Autodesk Inventor part; units mm, degrees
ref_plane "YZ Plane" through (0, 0, 0) normal (1, 0, 0) x (0, 1, 0)
ref_plane "XZ Plane" through (0, 0, 0) normal (0, 1, 0) x (-1, 0, 0)
ref_plane "XY Plane" through (0, 0, 0) normal (0, 0, 1) x (1, 0, 0)
ref_plane "Arbeitsebene1" through (-10.2983, 3.243, -1) normal (0, 0, -1) x (-1, 0, 0)
sketch "Skizze1" plane through (-10.2983, 3.243, -1) normal (0, 0, -1) x (-1, 0, 0)
  line L0 (2.7017, 34.757) -> (-23.2983, 34.757)
  line L1 (-23.2983, 34.757) -> (-23.2983, -41.243)
  line L2 (-23.2983, -41.243) -> (2.7017, -41.243)
  line L3 (2.7017, -41.243) -> (2.7017, 34.757)
  line L4 (3.7017, -42.243) -> (-24.2983, -42.243)
  line L5 (-24.2983, -42.243) -> (-24.2983, 35.757)
  line L6 (-24.2983, 35.757) -> (3.7017, 35.757)
  line L7 (3.7017, 35.757) -> (3.7017, -42.243)
  line L8 (7.7017, -46.243) -> (-28.2983, -46.243)
  line L9 (-28.2983, -46.243) -> (-28.2983, 39.757)
  line L10 (-28.2983, 39.757) -> (7.7017, 39.757)
  line L11 (7.7017, 39.757) -> (7.7017, -46.243)
  point P0 (-10.2983, -3.243)
  dimension "d1" = 4
  dimension "d39" = 36
extrude "Extrusion1" add sketch "Skizze1" along normal blind 3 contours L8 L9 L10 L11
sketch "Skizze2" plane through (-10.2983, 3.243, -1) normal (0, 0, 1) x (1, 0, 0)
  line L0 (24.2983, 35.757) -> (24.2983, -42.243)
  line L1 (24.2983, -42.243) -> (-3.7017, -42.243)
  line L2 (-3.7017, -42.243) -> (-3.7017, 35.757)
  line L3 (-3.7017, 35.757) -> (24.2983, 35.757)
  line L4 (-7.7017, -46.243) -> (28.2983, -46.243)
  line L5 (28.2983, -46.243) -> (28.2983, 39.757)
  line L6 (28.2983, 39.757) -> (-7.7017, 39.757)
  line L7 (-7.7017, 39.757) -> (-7.7017, -46.243)
  line L8 (22.2983, 33.757) -> (22.2983, -40.243)
  line L9 (22.2983, -40.243) -> (-1.7017, -40.243)
  line L10 (-1.7017, -40.243) -> (-1.7017, 33.757)
  line L11 (-1.7017, 33.757) -> (22.2983, 33.757)
  line L12 (21.2983, -39.243) -> (21.2983, 32.757)
  line L13 (21.2983, 32.757) -> (-0.7017, 32.757)
  line L14 (-0.7017, 32.757) -> (-0.7017, -39.243)
  line L15 (-0.7017, -39.243) -> (21.2983, -39.243)
  point P0 (10.2983, -3.243)
  dimension "d4" = 2
  dimension "d45" = 1
extrude "Extrusion2" add sketch "Skizze2" along normal blind 1 contours L0 L1 L2 L3 | L7 L6 L5 L4 | L8 L9 L10 L11
ref_plane "Arbeitsebene2" through (-18, -43, -2.5) normal (0, -1, 0) x (1, 0, 0)
sketch "Skizze9" plane through (-18, -43, -4) normal (-1, 0, 0) x (0, 0, 1)
  line L0 (0, 86) -> (4, 86)
  line L1 (0, 0) -> (0, 86)
  line L2 (4, 0) -> (0, 0)
  line L3 (4, 86) -> (4, 0)
  line L4 (4, 0) -> (3, 0)
  line L5 (3, 0) -> (3, 86)
  line L6 (3, 86) -> (4, 86)
  line L7 (4, 86) -> (4, 0)
  line L8 (4, 0) -> (3, 86) construction
  line L9 (3, 0) -> (4, 86) construction
  dimension "d27" = 1
extrude "Extrusion9" add sketch "Skizze9" along normal blind 3 contours L0 L3 L2 L5
sketch "Skizze10" plane through (18, -43, -4) normal (1, 0, 0) x (0, 0, -1)
  line L0 (-3, 86) -> (-3, 0)
  line L1 (-3, 0) -> (-4, 0)
  line L2 (-4, 0) -> (-4, 86)
  line L3 (-4, 86) -> (-3, 86)
  point P0 (-4, 43)
extrude "Extrusion10" add sketch "Skizze10" along normal blind 3
sketch "Skizze11" plane through (-10.2983, 3.243, 0) normal (0, 0, 1) x (1, 0, 0)
  line L0 (22.2983, -40.243) -> (-1.7017, -40.243)
  line L1 (-1.7017, -40.243) -> (-1.7017, 33.757)
  line L2 (-1.7017, 33.757) -> (22.2983, 33.757)
  line L3 (22.2983, 33.757) -> (22.2983, -40.243)
  line L4 (31.2983, 39.757) -> (-9.4351, 39.757)
  line L5 (-9.4351, 39.757) -> (-9.4351, 59.757)
  line L6 (-9.4351, 59.757) -> (31.2983, 59.757)
  line L7 (31.2983, 59.757) -> (31.2983, 39.757)
  line L8 (28.2983, 42.757) -> (-6.4351, 42.757)
  line L9 (-6.4351, 42.757) -> (-6.4351, 56.757)
  line L10 (-6.4351, 56.757) -> (28.2983, 56.757)
  line L11 (28.2983, 56.757) -> (28.2983, 42.757)
  point P0 (10.2983, -3.243)
  dimension "d32" = 20
  dimension "d33" = 3
extrude "Extrusion11" add sketch "Skizze11" against normal up to surface (4 mm away) contours L4 L5 L6 L7
sketch "Skizze12" plane through (-10.2983, 3.243, 0) normal (0, 0, 1) x (1, 0, 0)
  line L0 (28.2983, 56.757) -> (28.2983, 42.757)
  line L1 (28.2983, 42.757) -> (-6.4351, 42.757)
  line L2 (-6.4351, 42.757) -> (-6.4351, 56.757)
  line L3 (-6.4351, 56.757) -> (28.2983, 56.757)
  line L4 (31.2983, -46.243) -> (31.2983, 59.757)
  line L5 (31.2983, 59.757) -> (-9.4351, 59.757)
  line L6 (-9.4351, 59.757) -> (-9.4351, 39.757)
  line L7 (35.2983, 40.5388) -> (-14.7017, 40.5388)
  line L8 (-14.7017, 40.5388) -> (-14.7017, 42.757)
  line L9 (-14.7017, 42.757) -> (35.2983, 42.757)
  line L10 (35.2983, 42.757) -> (35.2983, 40.5388)
  line L11 (35.2983, 40.5388) -> (-14.7017, 42.757) construction
  line L12 (-14.7017, 40.5388) -> (35.2983, 42.757) construction
  line L13 (31.2983, -46.243) -> (-10.7017, -46.243)
  line L14 (-10.7017, 39.757) -> (-9.4351, 39.757)
  line L15 (-10.7017, -46.243) -> (-10.7017, 39.757)
  point P0 (10.2983, -3.243)
  point P1 (10.2983, 41.6479)
  dimension "d36" = 50
extrude "Extrusion12" add sketch "Skizze12" against normal blind 10 contours L9 L4 L7 L6 L1 | L9 L10 L7 L4 | L6 L7 L8 L9
sketch "Skizze13" plane through (-10.2983, 3.243, -4) normal (0, 0, -1) x (-1, 0, 0)
  line L0 (-24.2983, -42.243) -> (-24.2983, 35.757)
  line L1 (-24.2983, 35.757) -> (3.7017, 35.757)
  line L2 (3.7017, 35.757) -> (3.7017, -42.243)
  line L3 (3.7017, -42.243) -> (-24.2983, -42.243)
  line L4 (9.4351, 40.5388) -> (-31.2983, 40.5388)
  line L5 (-31.2983, 39.757) -> (-31.2983, 40.5388)
  line L6 (-28.2983, 39.757) -> (-31.2983, 39.757)
  line L7 (-28.2983, 39.757) -> (-28.2983, -46.243)
  line L8 (-28.2983, -46.243) -> (7.7017, -46.243)
  line L9 (7.7017, -46.243) -> (7.7017, 39.757)
  line L10 (9.4351, 39.757) -> (7.7017, 39.757)
  line L11 (9.4351, 40.5388) -> (9.4351, 39.757)
  line L12 (-27.2983, -42.243) -> (6.7017, -42.243)
  line L13 (6.7017, -42.243) -> (6.7017, 35.757)
  line L14 (6.7017, 35.757) -> (-27.2983, 35.757)
  line L15 (-27.2983, 35.757) -> (-27.2983, -42.243)
  line L16 (-27.2983, -42.243) -> (6.7017, 35.757) construction
  line L17 (6.7017, -42.243) -> (-27.2983, 35.757) construction
  point P0 (-10.2983, -3.243)
  dimension "d40" = 34
extrude "Extrusion13" cut sketch "Skizze13" against normal up to surface (3 mm away) contours L12 L15 L14 L0 | L2 L14 L13 L12
sketch "Skizze14" plane through (-10.2983, 3.243, -4) normal (0, 0, -1) x (-1, 0, 0)
  line L0 (6.7017, -42.243) -> (-27.2983, -42.243)
  line L1 (-27.2983, -42.243) -> (-27.2983, 35.757)
  line L2 (-27.2983, 35.757) -> (6.7017, 35.757)
  line L3 (6.7017, 35.757) -> (6.7017, -42.243)
  line L4 (9.4351, 40.5388) -> (-31.2983, 40.5388)
  line L5 (-31.2983, 39.757) -> (-31.2983, 40.5388)
  line L6 (-28.2983, 39.757) -> (-31.2983, 39.757)
  line L7 (-28.2983, 39.757) -> (-28.2983, -46.243)
  line L8 (-28.2983, -46.243) -> (7.7017, -46.243)
  line L9 (7.7017, -46.243) -> (7.7017, 39.757)
  line L10 (9.4351, 39.757) -> (7.7017, 39.757)
  line L11 (9.4351, 40.5388) -> (9.4351, 39.757)
  point P0 (-10.2983, -3.243)
extrude "Extrusion14" cut sketch "Skizze14" against normal blind 1
sketch "Skizze15" plane through (-10.2983, 3.243, -1) normal (0, 0, -1) x (-1, 0, 0)
  line L0 (0.7017, -39.243) -> (-21.2983, -39.243)
  line L1 (-21.2983, -39.243) -> (-21.2983, 32.757)
  line L2 (-21.2983, 32.757) -> (0.7017, 32.757)
  line L3 (0.7017, 32.757) -> (0.7017, -39.243)
  line L4 (-27.2983, -42.243) -> (6.7017, -42.243)
  line L5 (6.7017, -42.243) -> (6.7017, 35.757)
  line L6 (6.7017, 35.757) -> (-27.2983, 35.757)
  line L7 (-27.2983, 35.757) -> (-27.2983, -42.243)
  line L8 (6.7017, -39.243) -> (-27.2983, -39.243)
  line L9 (-27.2983, -39.243) -> (-27.2983, 32.757)
  line L10 (-27.2983, 32.757) -> (6.7017, 32.757)
  line L11 (6.7017, 32.757) -> (6.7017, -39.243)
  line L12 (6.7017, -39.243) -> (-27.2983, 32.757) construction
  line L13 (-27.2983, -39.243) -> (6.7017, 32.757) construction
  point P0 (-10.2983, -3.243)
extrude "Extrusion15" cut sketch "Skizze15" against normal through all contours L3 L10 L5 L8 | L8 L7 L10 L1
properties part number "41_Objektträger_Tray"
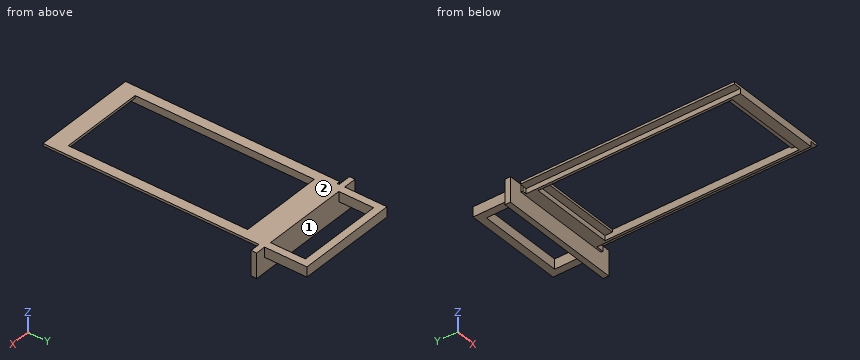
The listing builds one solid part. Answer for the finished solid, in the listing's coordinates (mm). Face numbers are marked on the shaded views. Coordinates: 2 decimals unless noted, no trailing zeros. Loops run counter-clockwise (first coordinate to the right, second up) from the corner with the lowest first, then second, coordinate; pieces in that order, holes last. Notation, with made-up numbers: M -0.5,59 L 58.5,59 A26 cw 58.5,82 Z; hole C 70,70 d1. An arc over 180 degrees is marked long. Answer in a Markdown table with one row per item.
1) Determine the mould class of the marked faces 1 and 2 for opening direction X: released by +X, released by -X, zero draft, split by the parting line, or undercut.
Answers below:
| item | result |
|---|---|
| face 1 | undercut |
| face 2 | zero draft |
2) Given pin 1 (1.1 mm diameter, centred on y = -11, z = -0.5, fed in from -X); pin 2 (0.5 mm diameter, centred on x = -19, z = -2, fed in from -Y); pin 3 (3.5 mm diameter, centred on x = -19.5, y = -3, fed in from -Z), each flat-ended and moving along its own axis, determine where each tip first touches the part or whether it passes through.
Answers below:
| item | result |
|---|---|
| pin 1 | x = -21 |
| pin 2 | y = 43 |
| pin 3 | z = -3 |
3) Find section A-A (y = -16). Determine the outline of the cut face in (x, z).
Answers below:
| item | result |
|---|---|
| outline | M -21,-1 L -18,-1 L -18,-3 L -17,-3 L -17,0 L -21,0 Z; M 17,-3 L 18,-3 L 18,-1 L 21,-1 L 21,0 L 17,0 Z |
4) Find section C-C (z = -2). Determine the outline of the cut face in (x, y).
Answers below:
| item | result |
|---|---|
| outline | M -25,43.78 L -19.73,43.78 L -19.73,43 L -18,43 L -18,-43 L 18,-43 L 18,43 L 21,43 L 21,43.78 L 25,43.78 L 25,46 L 21,46 L 21,63 L -19.73,63 L -19.73,46 L -25,46 Z; hole M -17,-39 L 17,-39 L 17,39 L -17,39 Z; hole M -16.73,46 L 18,46 L 18,60 L -16.73,60 Z |
5) Find the intervals of material crossed by probe 1 along Y at (x, z) = (-16, -2.5); probe 2 along Y at (x, z) = (17.5, -1.5); probe 3 along X at (y, z) = (0, -2), in increasing order.
Answers below:
| item | result |
|---|---|
| probe 1 | -43 to -39, 39 to 46, 60 to 63 |
| probe 2 | -43 to 46, 60 to 63 |
| probe 3 | -18 to -17, 17 to 18 |
6) Find section D-D (y = 55.5). Determine the outline of the cut face in (x, z), then the cut area to 3 significant figures.
Answers below:
| item | result |
|---|---|
| outline | M -19.73,-4 L -16.73,-4 L -16.73,0 L -19.73,0 Z; M 18,-4 L 21,-4 L 21,0 L 18,0 Z |
| area | 24.0 mm^2 |
7) Find section B-B (x = 7.5). Determine the outline of the cut face in (y, z), then the cut area to 3 significant figures.
Answers below:
| item | result |
|---|---|
| outline | M -43,-3 L -39,-3 L -39,-1 L -36,-1 L -36,0 L -43,0 Z; M 36,-1 L 39,-1 L 39,-3 L 43.78,-3 L 43.78,-10 L 46,-10 L 46,0 L 36,0 Z; M 60,-4 L 63,-4 L 63,0 L 60,0 Z |
| area | 66.5 mm^2 |
